Can you work these out from the model? Positions are in its coordinate system, mm. A direction names the side the tool comes from. Give positions to 0.01 mm unless a question says otherwise; leave off trailing zeros. Order: outer loops, then holes, each group sorted by start corner. A loop starts at its lowest first (then second) coordinate and runs counter-clockwise, first axis right, second up.
Item 1: I'm going to push flat-ended pins straight in: pin 1 Ø1.2 at (x, y) = (20, 23) entering from -Z; pin 2 Ø5 at (x, z) = (10, 4.5) entering from +Y. Where does each tip first touch, or does it pass through?
Item 2: If I drill on line 1 along Y through (x, z) = (20, 7.25) (3 decimals); line 2 along Y through (x, z) = (17.5, 4); line 3 along X through (y, z) = (15, 5.5), over which ranges is the centre line in solid material (lowest first)?
Item 3: Which directions (+Z, -Z, +X, -X, +Y, -Y) give clear straight access to the entire face, cutting with the end or side of a thin tool? Please do faces 1 (the flat face through (-16, 25, 5)), 2 (the flat face through (-23, 33, 5)), 3 (the flat face through (-18, 18, 5)).
Item 4: I want a section at D-D, the plane y = 23. Write out the boundary of the cut face in (x, z) (3 decimals), then the cut area to 3 significant figures.
Item 5: I want a section at B-B, the plane x = 0. Write out the boundary of the cut face in (y, z), then the cut area to 3 significant figures.
Item 6: I want a section at A-A, the plane y = 9. Write out the boundary of the cut face in (x, z).
Item 7: If we mould it in two halves opening along Y, with no side actions, what happens to faces 4 (the cylindrical face through (20.76, -14.31, 4.93)), 5 (the cylindrical face through (-6, 0, 5)), 6 (the flat face through (-30, 4, 5)), 7 (the flat face through (23, 33, 5))? For each: +Y half, -Y half, draft (parallel to the pull), parting line (faces both ways), or undercut.
Item 8: I want a section at C-C, the plane z = 8. Write out the boundary of the cut face in (x, y) (3 decimals), then the cut area to 3 significant figures.
```python
from build123d import *

# Parameters (mm, degrees)
SKETCH1_W                = 60
SKETCH1_H                = 58
SKETCH1_R                = 6
SKETCH1_W_2              = 42
SKETCH1_H_2              = 10
BOSS_EXTRUDE1_DEPTH      = 10
M2_5X0_45_TAPPED_HOLE1_D = 2.05
SKETCH4_W                = 32
SKETCH4_H                = 15
CUT_EXTRUDE1_DEPTH       = 11
CUT_EXTRUDE1_DEPTH_BACK  = 1


with BuildPart() as part:
    # Sketch1 → Boss-Extrude1 (new body)
    with BuildSketch(Plane.XY):
        with Locations((0, 4)):
            Rectangle(SKETCH1_W, SKETCH1_H)
        Circle(SKETCH1_R, mode=Mode.SUBTRACT)
        with Locations((0, 13)):
            Rectangle(SKETCH1_W_2, SKETCH1_H_2, mode=Mode.SUBTRACT)
        with Locations((0, 13)):
            Rectangle(SKETCH1_W_2, SKETCH1_H_2)
    extrude(amount=BOSS_EXTRUDE1_DEPTH)

    # M2.5x0.45 Tapped Hole1 (through all)
    with Locations(Plane.XY.offset(10)):
        with Locations((20, 23), (-20, 23), (-20, -15), (20, -15)):
            Hole(M2_5X0_45_TAPPED_HOLE1_D / 2)

    # Sketch4 → Cut-Extrude1 (cut, two sides)
    with BuildSketch(Plane.XY) as cut_extrude1_sk:
        with Locations((0, 25.5)):
            Rectangle(SKETCH4_W, SKETCH4_H)
        Polygon((16, 18), (-16, 18), (-21, 18), (-21, 8), (21, 8), (21, 18), align=None)
    extrude(amount=CUT_EXTRUDE1_DEPTH, mode=Mode.SUBTRACT)
    extrude(cut_extrude1_sk.sketch, amount=-CUT_EXTRUDE1_DEPTH_BACK, mode=Mode.SUBTRACT)


solid = part.part
```
Results list:
1. pin 1: passes through
1. pin 2: stops at y = 8
2. line 1: y = -25 to -16.025, -13.975 to 8, 18 to 21.975, 24.025 to 33
2. line 2: y = -25 to 8, 18 to 33
2. line 3: x = -30 to -21, 21 to 30
3. face 1: +Z, -Z, +Y
3. face 2: +Z, -Z, +X, -X, +Y
3. face 3: +Z, -Z
4. outline: (-30, 0) - (-21.025, 0) - (-21.025, 10) - (-30, 10) - close; (-18.975, 0) - (-16, 0) - (-16, 10) - (-18.975, 10) - close; (16, 0) - (18.975, 0) - (18.975, 10) - (16, 10) - close; (21.025, 0) - (30, 0) - (30, 10) - (21.025, 10) - close
4. area: 239 mm2
5. outline: (-25, 0) - (-6, 0) - (-6, 10) - (-25, 10) - close; (6, 0) - (8, 0) - (8, 10) - (6, 10) - close
5. area: 210 mm2
6. outline: (-30, 0) - (-21, 0) - (-21, 10) - (-30, 10) - close; (21, 0) - (30, 0) - (30, 10) - (21, 10) - close
7. face 4: undercut
7. face 5: undercut
7. face 6: draft
7. face 7: +Y half
8. outline: (-30, -25) - (30, -25) - (30, 33) - (16, 33) - (16, 18) - (21, 18) - (21, 8) - (-21, 8) - (-21, 18) - (-16, 18) - (-16, 33) - (-30, 33) - close; hole circle Ø2.05 at (-20, -15); hole circle Ø2.05 at (-20, 23); hole circle Ø12 at (0, 0); hole circle Ø2.05 at (20, -15); hole circle Ø2.05 at (20, 23)
8. area: 2,450 mm2
